from build123d import *

# Parameters (mm, degrees)
SALIENTE_EXTRUIR1_DEPTH      = 3
TALADRO_DE_MARGEN_PARA_M41_D = 4.5
REDONDEO1_R                  = 5


with BuildPart() as part:
    # Croquis1 → Saliente-Extruir1 (new, symmetric)
    with BuildSketch(Plane.XY):
        Polygon((0, 0), (0, 80), (30, 50), (30, 0), align=None)
    extrude(amount=SALIENTE_EXTRUIR1_DEPTH, both=True)

    # Taladro de margen para M41 (through all)
    with Locations(Plane.XY.offset(3)):
        with Locations((5, 5), (25, 5)):
            Hole(TALADRO_DE_MARGEN_PARA_M41_D / 2)

    # Redondeo1
    redondeo1_edges = [part.edges().sort_by_distance(p)[0] for p in [
        (0, 0, 0),
        (30, 50, 0),
        (30, 0, 0),
    ]]
    fillet(redondeo1_edges, radius=REDONDEO1_R)


solid = part.part
Geometry check sheet. Reference: the model listing, model coordinates, mm. Round coordinates to 2 decimals unless told otherwise and drop trailing zeros. Loops run counter-clockwise (first coordinate to the right, second up) from the corner with the lowest first, then second, coordinate; pieces in that order, holes last.
Item 1: Cross-section at C-C on y = 59. Record the boundary of the cut face in (x, z).
Item 2: Thickness scan on line 1 (Y direction, x = 25, z = 0.15); line 2 (Y direction, x = 24, z = 1.4); line 3 (Y direction, x = 8.5, z = 2.75). Record the ranges inside material, lowest first.
Item 3: Gauge pin test, flat ends, axial feed: pin 1 (1 mm diameter, centred on y = 68, z = 1.5, fed in from +X); pin 2 (1 mm diameter, centred on x = 5.5, z = 0.5, fed in from +Y). Record the tip position at first contact, or that the pin passes through.
Item 4: Cross-section at B-B on x = 10. Record the boundary of the cut face in (y, z), then the cut area to 3 significant figures.
Item 5: Mould release check, pull along X, two halves, no side actions. Record for faces 1 (the cylindrical face through (2.854, 5.676, -0.042)), 2 (the flat face through (30, 27, 0)), 3 (the cylindrical face through (1, 2, 0)): pulls with the +X half, pulls with the -X half, needs draft (parallel to the pull), parting line crosses it, or undercut.
Item 6: Cross-section at A-A on z = -0.4. Record the boundary of the cut face in (x, y), then the cut area to 3 significant figures.
Answer sheet:
1. outline: (0, -3) - (21, -3) - (21, 3) - (0, 3) - close
2. line 1: y = 0 to 2.75, 7.25 to 55
2. line 2: y = 0 to 2.98, 7.02 to 56
2. line 3: y = 0 to 71.5
3. pin 1: stops at x = 12.5
3. pin 2: stops at y = 75
4. outline: (0, -3) - (70, -3) - (70, 3) - (0, 3) - close
4. area: 420 mm2
5. face 1: undercut
5. face 2: pulls with the +X half
5. face 3: pulls with the -X half
6. outline: (0, 5) arc R5 ccw to (5, 0) - (25, 0) arc R5 ccw to (30, 5) - (30, 47.93) arc R5 ccw to (28.54, 51.46) - (0, 80) - close; hole circle Ø4.5 at (5, 5); hole circle Ø4.5 at (25, 5)
6. area: 1,910 mm2
